Print and shaded views of the part. All mm, measured from the part's lowest x, y and z. A direction names the side the tool comes from. Round coordinates to 2 decimals unless told otherwise and drop trailing zeros. Loops run counter-clockwise (first coordinate to the right, second up) from the corner with the lowest first, then second, coordinate; pieces in that order, holes last. Notation, with made-up numbers: (14.25, -4) - (60.25, -4) arc R15 ccw to (60.25, 24) - close; hole circle Ø8 at (-9, 63.5). An arc over 180 degrees is marked (long way). Answer as a JSON object with one key per item and string values.
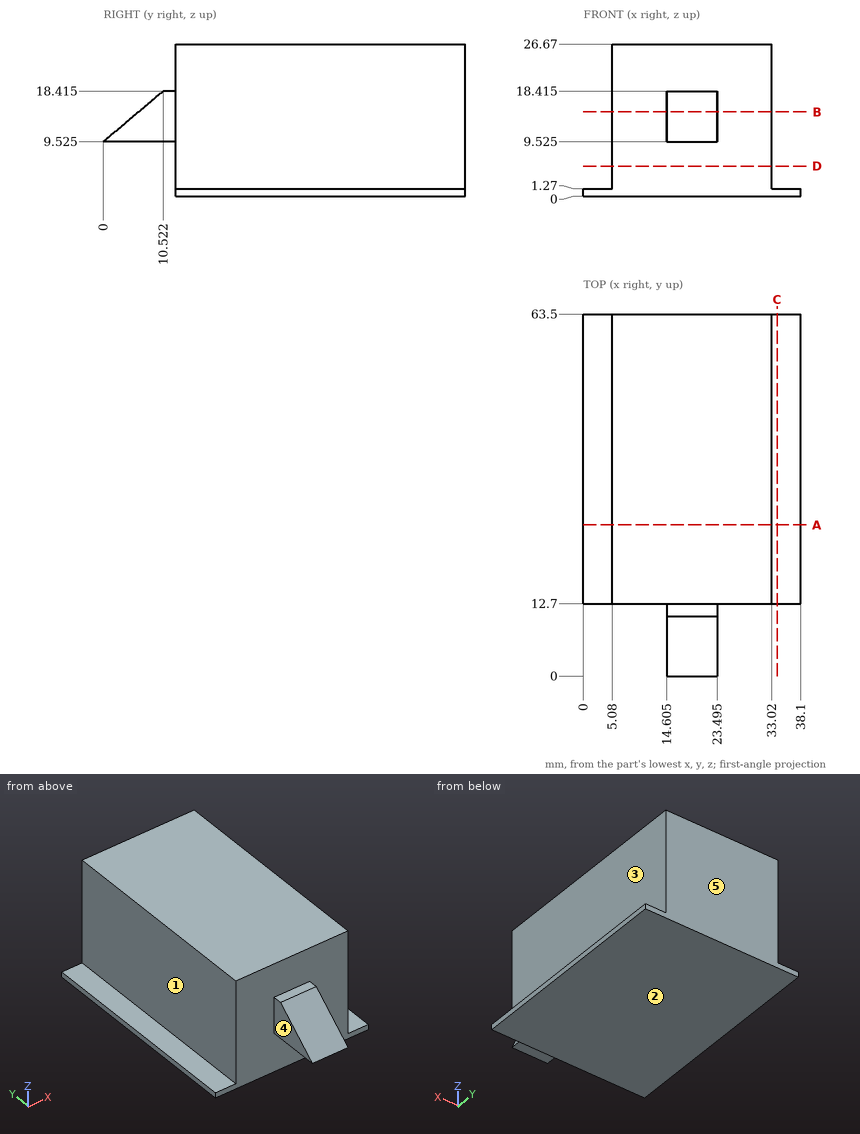
1) Probe probe 1 along Y at (x, z) = (25.5, 18.5); probe 2 along X at (y, z) = (43.5, 9); probe 3 along X at (y, z) = (11, 13.5) (1 decimal). List the from-to ranges inside material, lowest first.
Values follow:
{"probe 1": "12.7 to 63.5", "probe 2": "5.08 to 33.02", "probe 3": "14.6 to 23.5"}
2) Slice it at D-D on z = 5.25. List the corners of the cut face in (x, y), then the cut area to 3 significant figures.
Values follow:
{"outline": "(5.08, 12.7) - (33.02, 12.7) - (33.02, 63.5) - (5.08, 63.5) - close", "area": "1,420 mm²"}
3) Slice it at C-C on x = 34. List the corners of the cut face in (y, z).
Values follow:
{"outline": "(12.7, 0) - (63.5, 0) - (63.5, 1.27) - (12.7, 1.27) - close"}
4) Drop flat-ended pins along their axis: P1, Ø4, axis at x = 24, z = 20.5, coming from the -Y side; P2, Ø7.5, axis at y = 30.5, z = 15.5, coming from the +X side; P3, Ø8, axis at x = 26, z = 11.5, coming from the -Y side; P4, Ø4.5, axis at x = 19, y = 6.5, coming from the -Z side (3 decimals). Give the stop position or say it passes through.
Values follow:
{"P1": "y = 12.7", "P2": "x = 33.02", "P3": "y = 0", "P4": "z = 9.525"}
5) Slice it at B-B on z = 14.75. List the corners of the cut face in (x, y) (1 decimal), then the cut area to 3 significant figures.
Values follow:
{"outline": "(5.1, 12.7) - (14.6, 12.7) - (14.6, 6.2) - (23.5, 6.2) - (23.5, 12.7) - (33, 12.7) - (33, 63.5) - (5.1, 63.5) - close", "area": "1,480 mm²"}
6) Slice it at A-A on y = 26.5. List the corners of the cut face in (x, z).
Values follow:
{"outline": "(0, 0) - (38.1, 0) - (38.1, 1.27) - (33.02, 1.27) - (33.02, 26.67) - (5.08, 26.67) - (5.08, 1.27) - (0, 1.27) - close"}
7) Tool access for the marked faces 1, 2, 3, 4 and 5: list every direction of +Z, -Z, +X, -X, +Y, -Y with a clear straight run to the whole face (end or side of a thin tool).
Values follow:
{"face 1": "+Z, -X, +Y, -Y", "face 2": "-Z, +X, -X, +Y, -Y", "face 3": "+Z, +X, +Y, -Y", "face 4": "+Z, -Z, -X, -Y", "face 5": "+Z, -Z, +X, -X, +Y"}
